For this review, use the dimensioned drawing (mm, ordinates from the lowest corner) and the shaded views. Give positions to 0.01 mm unless a question says otherwise; leave off trailing zeros. Write each loop counter-clockwise with the first axis right and the second up, starting at its lowest first coordinate (ties: lowest second). Pieces come first, ordered by that corner, then holes. Notation, with made-up numbers: M -28.5,55 L -22.5,55 A25 ccw -22.5,91 Z; hole C 18,-27.75 d9. An arc over 180 degrees is marked long. Answer in a Markdown table with one row per item.
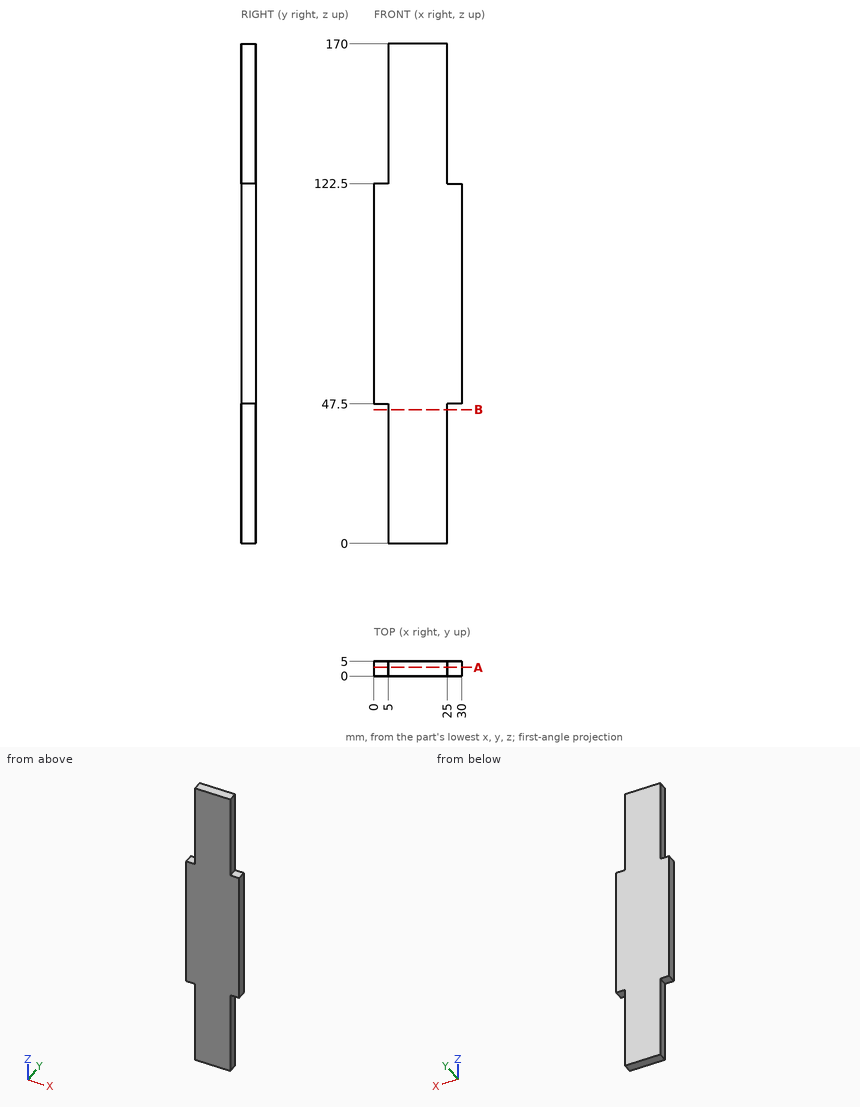
1) Add section A-A (y = 2.95). Write out the cut boundary in (x, z).
Geometry says:
| item | result |
|---|---|
| outline | M 0,47.5 L 5,47.5 L 5,0 L 25,0 L 25,47.5 L 30,47.5 L 30,122.5 L 25,122.5 L 25,170 L 5,170 L 5,122.5 L 0,122.5 Z |
2) Add section B-B (z = 45.5). Write out the cut boundary in (x, y).
Geometry says:
| item | result |
|---|---|
| outline | M 5,0 L 25,0 L 25,5 L 5,5 Z |
3) Insertion check: P1, Ø2.5, axis at y = 1.5, z = 16, coming from the +X side; P2, Ø2.5, axis at x = 2, y = 2, coming from the -Z side. Each pin has a flat end and moves straight along its axis. Give the tip position at first contact, or say it passes through.
Geometry says:
| item | result |
|---|---|
| P1 | x = 25 |
| P2 | z = 47.5 |
4) To check wall thickness, follow probe 1 along X at (y, z) = (0.9, 39.5); probe 2 along Z at (x, y) = (26.25, 1.05). State the ranges of each line that lie inside material, in increasing order. Write a range as [from, to].
Geometry says:
| item | result |
|---|---|
| probe 1 | [5, 25] |
| probe 2 | [47.5, 122.5] |
